```python
from build123d import *

# Parameters (mm, degrees)
SKETCH1_R           = 400
BOSS_EXTRUDE1_DEPTH = 10
SKETCH2_R           = 20
CUT_EXTRUDE2_DEPTH  = 5


with BuildPart() as part:
    # Sketch1 → Boss-Extrude1 (new body)
    with BuildSketch(Plane(origin=(0, 0, 0), x_dir=(1, 0, 0), z_dir=(0, 1, 0))):
        with Locations(Location((0, 0, 0), (0, 0, 270))):
            Circle(SKETCH1_R)
    extrude(amount=BOSS_EXTRUDE1_DEPTH)

    # Sketch2 → Cut-Extrude2 (cut)
    with BuildSketch(Plane(origin=(0, 10, 0), x_dir=(1, 0, 0), z_dir=(0, 1, 0))):
        with Locations(Location((360, 0, 0), (0, 0, 270))):
            Circle(SKETCH2_R)
        with Locations(Location((-360, 0, 0), (0, 0, 270))):
            Circle(SKETCH2_R)
        with Locations(Location((0, 360, 0), (0, 0, 270))):
            Circle(SKETCH2_R)
    extrude(amount=-CUT_EXTRUDE2_DEPTH, mode=Mode.SUBTRACT)


solid = part.part
```
CAD build for the part. Positions are in the model's coordinates, mm. A direction names the side the tool comes from. Give positions to 0.01 mm unless a question says otherwise; leave off trailing zeros. Order: outer loops, then holes, each group sorted by start corner. A loop starts at its lowest first (then second) coordinate and runs counter-clockwise, first axis right, second up. Notation, with made-up numbers: M 76.25,39.5 L 89.25,39.5 A15 cw 89.25,49.5 Z; hole C -7,-40 d4. An arc over 180 degrees is marked long. Put each result on its own line as item: value. Start each with the question number.
(1) Flat gauge pins, fed straight in: pin 1 Ø5 at (y, z) = (5, 257.5) entering from +X; pin 2 Ø24 at (x, z) = (360, 0) entering from +Y; pin 3 Ø2 at (x, y) = (-145, 5) entering from -Z. Where does each tip first touch, or does it go through?
(2) Saw through at C-C, the plane y = 7.75. Write the cut outline in (x, z).
(3) Saw through at D-D, the plane x = -360. Write the cut outline in (y, z), then the cut area to 3 significant figures.
(4) Mould opens along Z. For faces 3 (the cylindrical face through (120.15, 4.93, 381.53)), 4 (the cylindrical face through (-7.66, 7.535, -341.525)), 5 (the flat face through (6, 0, -6)) say: +Z half, -Z half, draft (parallel to the pull), parting line (faces both ways), or undercut.
(5) Which spindle directions (+Z, -Z, +X, -X, +Y, -Y) get a long thin tool onto all of the face, cutting with end or side? Do faces 1 (the cylindrical face through (340.476, 7.535, -4.336)), 2 (the flat face through (6, 10, -6)). Say none if no direction does.
(6) Saw through at B-B, the plane z = 0. Write the cut outline in (x, y), then the cut area to 3 significant figures.
(7) Saw through at A-A, the plane x = 0. Write the cut outline in (y, z), then the cut area to 3 significant figures.
(8) Drill centre lines: line 1 along X through (y, z) = (6.5, 0); line 2 along X through (y, z) = (8.25, 12.5); line 3 along Z through (x, y) = (-7.5, 9). Where is each one in solid material? Low to high.
Check result:
1. pin 1: stops at x = 308.18
1. pin 2: stops at y = 5
1. pin 3: stops at z = -373.18
2. outline: C 0,0 d800; hole C -360,0 d40; hole C 0,-360 d40; hole C 360,0 d40
3. outline: M 0,-174.36 L 10,-174.36 L 10,-20 L 5,-20 L 5,20 L 10,20 L 10,174.36 L 0,174.36 Z
3. area: 3,290 mm2
4. face 3: parting line
4. face 4: undercut
4. face 5: draft
5. face 1: +Y
5. face 2: +Z, -Z, +X, -X, +Y
6. outline: M -400,0 L 400,0 L 400,10 L 380,10 L 380,5 L 340,5 L 340,10 L -340,10 L -340,5 L -380,5 L -380,10 L -400,10 Z
6. area: 7,600 mm2
7. outline: M 0,-400 L 10,-400 L 10,-380 L 5,-380 L 5,-340 L 10,-340 L 10,400 L 0,400 Z
7. area: 7,800 mm2
8. line 1: x = -400 to -380, -340 to 340, 380 to 400
8. line 2: x = -399.8 to -375.61, -344.39 to 344.39, 375.61 to 399.8
8. line 3: z = -399.93 to -378.54, -341.46 to 399.93
